Verification items for the finished model (mm, model axes). Face numbers are marked on the shaded views. A direction names the side the tool comes from. Coordinates: 2 decimals unless noted, no trailing zeros. Order: outer loops, then holes, each group sorted by start corner. A loop starts at its lowest first (then second) coordinate and runs counter-clockwise, first axis right, second up. Notation, with made-up numbers: M 38.25,28.5 L 75.25,28.5 A21 ccw 75.25,47.5 Z; hole C -30.75,59 d6. An arc over 180 degrees is marked long. Answer as a JSON object with one key per item and string values. Group by question number.
(1) Access from +Z, -Z, +X, -X, +Y, -Y to the whole of each face (thin tool, end or side, straight path). Record for the marked faces 1, 2 and 3.
(2) Mould release check, pull along X, two halves, no side actions. Record for the marked faces 4, 5 and 6: released by +X, released by -X, zero draft, split by the parting line, or undercut.
(3) Cross-section at C-C (y = 0). Count the separate pieces of the cut face and the enclosed holes in it, plus the area to 3 significant figures.
(4) Cross-section at D-D (z = 7.5). Enter the section's corners in (x, y) (3 decimals), plus the area to 3 significant figures.
(5) Material ranges on line 1 (X direction, y = 0, z = 2.5) (3 decimals); line 2 (X direction, y = 1.5, z = 0.75); line 3 (X direction, y = 0, z = 9.25) (3 decimals), recorded low to high.
(6) Cross-section at B-B (x = 6.5). Enter the section's corners in (y, z).
(7) Gauge pin test, flat ends, axial feed: pin 1 Ø2.5 at (x, y) = (0, 0.5) entering from +Z; pin 2 Ø4.5 at (x, y) = (14, 0.5) entering from +Z; pin 3 Ø2 at (y, z) = (2.5, 9) entering from -X; pin 4 Ø3 at (x, y) = (14.5, -0.5) entering from -Z. Record the tip position at first contact, or that the pin passes through.
(8) Cross-section at A-A (z = 1.5). Enter the section's corners in (x, y) (3 decimals).
Autodesk Fusion 360 part; units mm, degrees
sketch "Sketch1" plane through (0, 0, 0) normal (0, 0, 1) x (1, 0, 0)
  circle A0 centre (0, 0) radius 1.525
  circle A1 centre (0, 0) radius 4.5
  circle A2 centre (13.2, 0) radius 1.525
  circle A3 centre (0, 0) radius 2.75
  circle A4 centre (13.2, 0) radius 2.75
  line L0 (0, 4.5) -> (13.2, 4.5)
  line L1 (13.2, -4.5) -> (0, -4.5)
  arc A5 (13.2, -4.5) -> (13.2, 4.5) centre (13.2, 0) ccw
  dimension "d1" = 3.05
  dimension "d2" = 9
  dimension "d3" = 9
  dimension "d4" = 3.05
  dimension "d5" = 5.5
  dimension "d6" = 5.5
  dimension "d7" = 13.2
extrude "Extrude1" add sketch "Sketch1" along normal blind 14 contours A1 | A3
extrude "Extrude2" add sketch "Sketch1" along normal blind 4.5 contours A1 L0 L1 A5 | A4
sketch "Sketch2" plane through (0, 0, 14) normal (0, 0, 1) x (-1, 0, 0)
  circle A0 centre (0, 0) radius 1.525
  circle A1 centre (0, 0) radius 4.5
  circle A2 centre (0, 0) radius 2.05
  dimension "d12" = 4.1
extrude "Extrude3" add sketch "Sketch2" along normal blind 1 contours A2
chamfer "Chamfer1" distance 1 angle 45 1 edges at (1.9113, -0.7413, 14)
sketch "Sketch3" plane through (0, 0, 4.5) normal (0, 0, 1) x (-1, 0, 0)
  circle A0 centre (-13.2, 0) radius 1.525
  line L0 (0, 4.5) -> (-13.2, 4.5)
  arc A1 (-13.2, 4.5) -> (-13.2, -4.5) centre (-13.2, 0) ccw
  line L1 (-13.2, -4.5) -> (0, -4.5)
  arc A2 (0, 4.5) -> (0, -4.5) centre (0, 0) ccw
  circle A3 centre (-13.2, 0) radius 2.05
  dimension "d16" = 4.1
extrude "Extrude4" add sketch "Sketch3" along normal blind 1 contours A3
chamfer "Chamfer2" distance 1 angle 45 1 edges at (15.1113, -0.7413, 4.5)
extrude "Extrude5" cut sketch "Sketch1" along normal blind 1 contours A3 | A4
chamfer "Chamfer3" distance 0.5 angle 45 10 edges at (6.6, -4.5, 0) (17.7, 0, 0) (6.6, 4.5, 0) (-4.5, 0, 0) (10.6361, -0.9944, 0) (-2.5639, -0.9944, 0) (-4.1955, -1.6273, 14) (6.6, -4.5, 4.5) (17.7, 0, 4.5) (6.6, 4.5, 4.5)
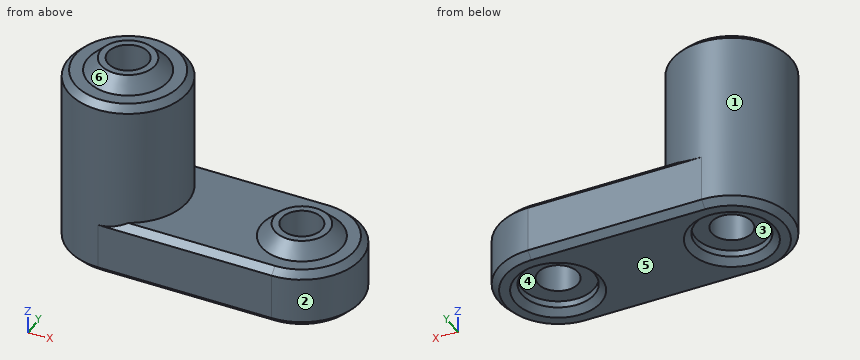
Taken from the geometry:
{
 "1": {"face 1": "+Z", "face 2": "+Z, -Z, +X", "face 3": "-Z"},
 "2": {"face 4": "undercut", "face 5": "zero draft", "face 6": "split by the parting line"},
 "3": {"separate pieces": "3", "enclosed holes": "0", "area": "127 mm²"},
 "4": {"outline": "C 0,0 d9; hole C 0,0 d3.05", "area": "56.3 mm²"},
 "5": {"line 1": "x = -4.5 to -1.525, 1.525 to 11.675, 14.725 to 17.7", "line 2": "x = -4.24 to -2.3, 2.3 to 10.9, 15.5 to 17.44", "line 3": "x = -4.5 to -1.525, 1.525 to 4.5"},
 "6": {"outline": "M -4.5,0.5 L -4,0 L 4,0 L 4.5,0.5 L 4.5,4 L 4,4.5 L -4,4.5 L -4.5,4 Z"},
 "7": {"pin 1": "stops at z = 15", "pin 2": "stops at z = 5.5", "pin 3": "stops at x = -4.24", "pin 4": "stops at z = 0.36"},
 "8": {"outline": "M 0,-4.5 L 13.2,-4.5 A4.5 ccw 13.2,4.5 L 0,4.5 A4.5 ccw Z; hole C 0,0 d3.05; hole C 13.2,0 d3.05"}
}
